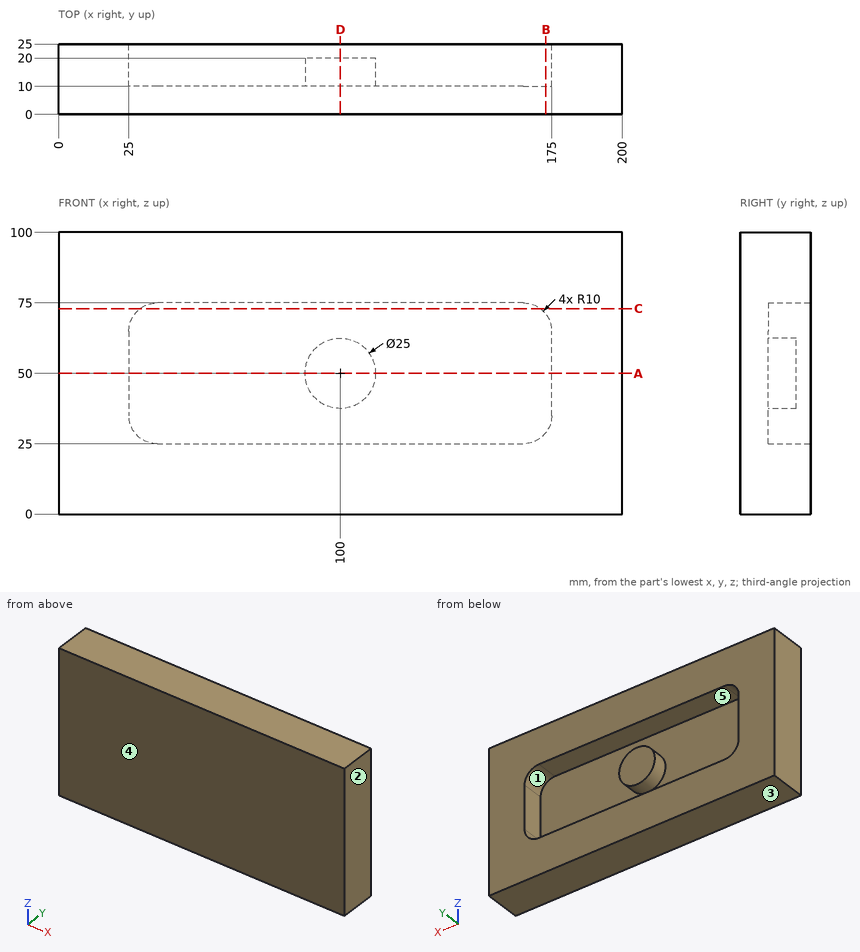
Here's the drawing with two shaded views (mm, measured from the low corner). I have some questions. A direction names the side the tool comes from. Round coordinates to 2 decimals unless told otherwise and drop trailing zeros. Loops run counter-clockwise (first coordinate to the right, second up) from the corner with the lowest first, then second, coordinate; pieces in that order, holes last. Notation, with made-up numbers: (73, -10) -> (111, -10) arc R29 cw to (111, 16) -> close; hole circle Ø5 at (82.25, 0.25). An arc over 180 degrees is marked (long way). Answer as CSV lines item,"result". Start each with the question number.
1. Imagine slicing it at C-C on z = 73. Write out the boundary of the cut face in (x, y).
2. Imagine slicing it at D-D on x = 100. Write out the boundary of the cut face in (y, z).
3. Imagine slicing it at A-A on z = 50. Write out the boundary of the cut face in (x, y).
4. For the marked faces 4 and 5, which set-ups out of +Z, -Z, +X, -X, +Y, -Y let a thin tool reach every point of the face, with its end or its side?
5. Imagine slicing it at B-B on x = 173. Write out the boundary of the cut face in (y, z).
6. I'm going to push a flat-ended pin straight in: P1, Ø15, axis at x = 101.5, z = 57.5, coming from the +Y side. Where does the tip first touch, or does it pass through?
7. I need wall thicknesses on probe 1 along Z at (x, y) = (59, 23.25); probe 2 along Z at (x, y) = (93, 16); probe 3 along X at (y, z) = (18.5, 58). Which ranges of each line are inside material? Lowest first, please. Write a range as from..to.
8. If we mould it in two halves opening along X, with no side actions, what happens to the marked faces 1, 2 and 3? For each: pulls with the +X half, pulls with the -X half, needs draft (parallel to the pull), parting line crosses it, or undercut.
Solution:
1,outline,"(0, 0) -> (200, 0) -> (200, 25) -> (171, 25) -> (171, 10) -> (29, 10) -> (29, 25) -> (0, 25) -> close"
2,outline,"(0, 0) -> (25, 0) -> (25, 25) -> (10, 25) -> (10, 37.5) -> (20, 37.5) -> (20, 62.5) -> (10, 62.5) -> (10, 75) -> (25, 75) -> (25, 100) -> (0, 100) -> close"
3,outline,"(0, 0) -> (200, 0) -> (200, 25) -> (175, 25) -> (175, 10) -> (112.5, 10) -> (112.5, 20) -> (87.5, 20) -> (87.5, 10) -> (25, 10) -> (25, 25) -> (0, 25) -> close"
4,face 4,"+Z, -Z, +X, -X, -Y"
4,face 5,"+Y"
5,outline,"(0, 0) -> (25, 0) -> (25, 29) -> (10, 29) -> (10, 71) -> (25, 71) -> (25, 100) -> (0, 100) -> close"
6,P1,"y = 20"
7,probe 1,"0..25, 75..100"
7,probe 2,"0..25, 39.64..60.36, 75..100"
7,probe 3,"0..25, 90.4..109.6, 175..200"
8,face 1,"undercut"
8,face 2,"pulls with the +X half"
8,face 3,"needs draft"
